```python
from build123d import *

# Parameters (mm, degrees)
SKETCH_1_R      = 35.893803705
EXTRUDE_1_DEPTH = 1.2
SHELL_1_T       = -0.5


with BuildPart() as part:
    # 스케치1 → 보스-돌출1 (new body)
    with BuildSketch(Plane(origin=(0, 0, 0), x_dir=(1, 0, 0), z_dir=(0, 1, 0))):
        with Locations(Location((0, 0, 0), (0, 0, 270))):
            Circle(SKETCH_1_R)
    extrude_1 = extrude(amount=EXTRUDE_1_DEPTH)

    # 스케치4 → 회전1 (revolve)
    with BuildSketch(Plane(origin=(0, 0, 0), x_dir=(0, 0, -1), z_dir=(1, 0, 0))):
        Polygon((-35.893803705, 2.7), (-35.893803705, 1.2), (0, 1.2), (0, 9), (-27.584076439, 9), (-27.584076439, 7.504385483), (-29.661508256, 8.553289112), (-29.661508256, 7.053289112), (-29.661508256, 5.553289112), (-31.738940072, 6.602192742), (-31.738940072, 5.102192742), (-31.738940072, 3.602192742), (-33.816371888, 4.651096371), (-33.816371888, 3.151096371), (-33.816371888, 1.651096371), align=None)
    revolve_1 = revolve(axis=Axis((0, 9, 0), (0, -1, 0)))

    # 대칭 복사1: 보스-돌출1, 회전1 across plane
    add(extrude_1.mirror(Plane(origin=(0, 9, 0), x_dir=(0, 0, 1), z_dir=(0, -1, 0))))
    add(revolve_1.mirror(Plane(origin=(0, 9, 0), x_dir=(0, 0, 1), z_dir=(0, -1, 0))))

    # 쉘1
    shell_1_openings = [part.faces().sort_by_distance(p)[0] for p in [
        (0, 18, 0),
        (0, 0, 0),
    ]]
    offset(amount=SHELL_1_T, openings=shell_1_openings, kind=Kind.INTERSECTION)


solid = part.part
```
The model under review builds one solid part; all positions refer to its coordinate system, in mm. Round coordinates to 2 decimals unless told otherwise and drop trailing zeros. Put each result on its own line as item: value.
Q1. Mouldability with a two-part tool opening along Y and no side actions: class faces 1 (the cylindrical face through (16.784, 9.021, -21.89)), 2 (the cylindrical face through (26.44, 9.03, -5.87)) as released by +Y, released by -Y, zero draft, split by the parting line, or undercut.
Result set:
face 1: undercut
face 2: zero draft
Q2. For pin 1 (8 mm diameter, centred on x = 14, y = 9.5, fed in from -Z); pin 2 (5 mm diameter, centred on y = 3, z = -26, fed in from -X); pin 3 (4 mm diameter, centred on x = -4, y = 10, fed in from +Z), all flat-tipped, find the tip position at first contact; note any pin that passes through.
Result set:
pin 1: stops at z = -31.25
pin 2: stops at x = -27.12
pin 3: stops at z = 31.63
Q3. To check wall thickness, follow L1, parallel to X at y = 14.55, z = 0; L2, parallel to Z at x = 8.5, y = 10; L3, parallel to X at y = 0.5, z = 0. State the ranges of each line that lie inside material, in increasing order.
Result set:
L1: x = -33.82 to -33.32, -32.55 to -31.24, 31.24 to 32.55, 33.32 to 33.82
L2: z = -28.42 to -27.27, -26.24 to -25.72, 25.72 to 26.24, 27.27 to 28.42
L3: x = -35.89 to -35.39, 35.39 to 35.89
